Part model, mm, in its own coordinate system. Round coordinates to 2 decimals unless told otherwise and drop trailing zeros. Write each loop counter-clockwise with the first axis right and the second up, starting at its lowest first coordinate (ties: lowest second). Pieces come first, ordered by that corner, then holes. Notation, with made-up numbers: M 85,-14.5 L 142,-14.5 A6 ccw 142,-10.5 Z; hole C 30,-14 d8. An arc over 180 degrees is marked long. Use one line per item in the form item = value. Start each with the question number.
Item 1: Cut at B-B, the plane z = 35.5. Give the cut face in (x, y).
Item 2: Probe L1, parallel to Y at x = 10, z = 26.5; L2, parallel to X at y = 34, z = 5; L3, parallel to X at y = 26, z = 7.5. List the from-to ranges inside material, lowest first.
Item 3: Cut at C-C, the plane x = 3. Give the cut face in (y, z).
Item 4: Flat gauge pins, fed straight in: pin 1 Ø1.5 at (y, z) = (35, 33) entering from +X; pin 2 Ø12 at (x, y) = (11, 18.5) entering from -Z; pin 3 Ø5 at (y, z) = (19, 6) entering from -X; pin 4 Ø10 at (y, z) = (15.5, 22) entering from -X. Where does each tip first touch, or does it go through?
Item 5: Cut at A-A, the plane y = 31. Give the cut face in (x, z), then the cut area to 3 significant figures.
Item 6: Cut at D-D, the plane y = 14. Give the cut face in (x, z).
from build123d import *

# Parameters (mm, degrees)
SKETCH1_W           = 40
SKETCH1_H           = 40
BOSS_EXTRUDE1_DEPTH = 40
CUT_EXTRUDE1_DEPTH  = 40
CUT_EXTRUDE2_DEPTH  = 40


with BuildPart() as part:
    # Sketch1 → Boss-Extrude1 (new body)
    with BuildSketch(Plane.XY):
        with Locations((20, 20)):
            Rectangle(SKETCH1_W, SKETCH1_H)
    extrude(amount=BOSS_EXTRUDE1_DEPTH)

    # Sketch2 → Cut-Extrude1 (cut)
    with BuildSketch(Plane.XY.offset(40)):
        Polygon((0, 0), (20, 40), (0, 40), align=None)
    extrude(amount=-CUT_EXTRUDE1_DEPTH, mode=Mode.SUBTRACT)

    # Sketch3 → Cut-Extrude2 (cut)
    with BuildSketch(Plane(origin=(0, 40, 0), x_dir=(1, 0, 0), z_dir=(0, 1, 0))):
        Polygon((20, -40), (40, -20), (40, -40), align=None)
    extrude(amount=-CUT_EXTRUDE2_DEPTH, mode=Mode.SUBTRACT)


solid = part.part
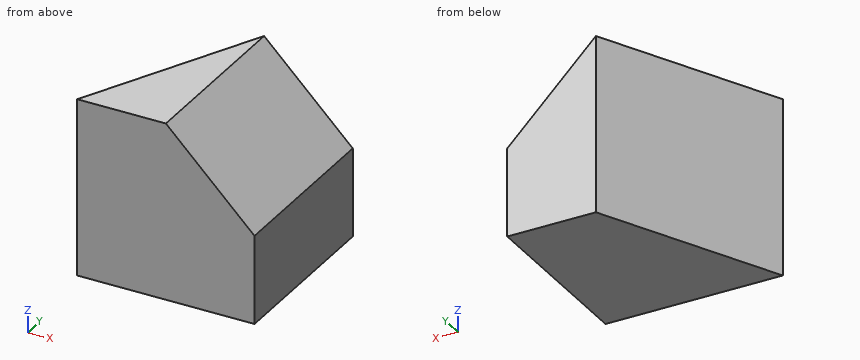
Model answer:
q1.outline = M 0,0 L 24.5,0 L 24.5,40 L 20,40 Z
q2.L1 = 0 to 20
q2.L2 = 17 to 40
q2.L3 = 13 to 40
q3.outline = M 0,0 L 6,0 L 6,40 L 0,40 Z
q4.pin_1 = 27.75
q4.pin_2 = 0
q4.pin_3 = 8.25
q4.pin_4 = 5.25
q5.outline = M 15.5,0 L 40,0 L 40,20 L 20,40 L 15.5,40 Z
q5.area = 780 mm²
q6.outline = M 7,0 L 40,0 L 40,20 L 20,40 L 7,40 Z
